Solid Edge part; units mm, degrees
sketch "Sketch1" plane through (10.8674, 10.8674, 0) normal (0, 0, 1) x (1, 0, 0)
  line L0 (-17.7956, -10.8674) -> (-14.3315, -4.8674)
  line L1 (-14.3315, -4.8674) -> (-7.4033, -4.8674)
  line L2 (-7.4033, -4.8674) -> (-3.9392, -10.8674)
  line L3 (-3.9392, -10.8674) -> (-7.4033, -16.8674)
  line L4 (-7.4033, -16.8674) -> (-14.3315, -16.8674)
  line L5 (-14.3315, -16.8674) -> (-17.7956, -10.8674)
extrude "Protrusion1" add sketch "Sketch1" along normal mid plane 3.2
sketch "Sketch2" plane through (0, 8.3963, 8.3963) normal (1, 0, 0) x (0, 1, 0)
  line L0 (-14.3963, -6.7963) -> (-17.1675, -8.3963)
  line L1 (-17.1675, -8.3963) -> (-14.3963, -9.9963)
revolve "RevolvedCutout1" cut sketch "Sketch2" angle 360 about axis through (0, 0, 1.6) along (0, 0, -1) material side at (0, -7.4106, 0.8433)
hole "Hål_M10" at (0, 0, 1.6) direction (0, 0, -1) diameter 8.376 end up to next
properties material "Iron"
The listing builds one solid part. Answer for the finished solid, in the listing's coordinates (mm). Coordinates: 2 decimals unless noted, no trailing zeros. Order: outer loops, then holes, each group sorted by start corner. A loop starts at its lowest first (then second) coordinate and runs counter-clockwise, first axis right, second up. Notation, with made-up numbers: (-25.5, 79.5) -> (20.5, 79.5) arc R10 cw to (20.5, 89.5) -> close; hole circle Ø4 at (38, -6.5). An arc over 180 degrees is marked (long way). Answer in a Markdown table with one row per item. Add a question column.
Item 1: Find section A-A (z = -0.3). Write down the section's boundary in (x, y), then the cut area to 3 significant figures.
Item 2: Find the intervals of material crossed by L1, parallel to Y at x = 0, z = -0.35; L2, parallel to Y at x = 3.25, z = -1.25; L3, parallel to X at y = -2.25, z = 1.3, in increasing order. Write a range as from..to.
Item 3: Determine the mould class of faces 1 (the face through (2.83, 3.087, 0.022)), 2 (the face through (-5.22, 2.96, -0.02)), 3 (the face through (-3, -4, 1.6)) for opening direction X: +X half, -X half, draft (parallel to the pull), parting line (faces both ways), or undercut.
Item 4: Each of these flat-tipped pins is pushed along its axis until it touches: P1, Ø5, axis at x = 0, y = 0, coming from the -Z side; P2, Ø1.5, axis at y = -3.5, z = 0.5, coming from the +X side. Where does it stop, or does it pass through?
Result set:
| question | item | result |
|---|---|---|
| 1 | outline | (-6.93, 0) -> (-3.46, -6) -> (3.46, -6) -> (6.93, 0) -> (3.46, 6) -> (-3.46, 6) -> close; hole circle Ø8.38 at (0, 0) |
| 1 | area | 69.6 mm² |
| 2 | L1 | y = -6..-4.19, 4.19..6 |
| 2 | L2 | y = -5.75..-2.64, 2.64..5.75 |
| 2 | L3 | x = -5.63..-3.53, 3.53..5.63 |
| 3 | face 1 | undercut |
| 3 | face 2 | -X half |
| 3 | face 3 | draft |
| 4 | P1 | passes through |
| 4 | P2 | stops at x = 5.34 |
